```python
from build123d import *

# Parameters (mm, degrees)
BOSS_EXTRUDE1_DEPTH         = 12.7
BOSS_EXTRUDE1_DEPTH_BACK    = 12.7
SKETCH3_R                   = 69.85
SKETCH3_R_2                 = 57.15
CUT_EXTRUDE1_DEPTH          = 102.996102867
TAP_DRILL_FOR_1_4_20_TAP1_D = 5.1054
FILLET1_R                   = 2.54


with BuildPart() as part:
    # Sketch3 → Boss-Extrude1 (new, two sides: drawn at the far end of the back side and taken through both)
    with BuildSketch(Plane.XY.offset(-BOSS_EXTRUDE1_DEPTH_BACK)):
        Circle(SKETCH3_R)
        Circle(SKETCH3_R_2, mode=Mode.SUBTRACT)
    extrude(amount=BOSS_EXTRUDE1_DEPTH + BOSS_EXTRUDE1_DEPTH_BACK)

    # Sketch4 → Cut-Extrude1 (cut, through all)
    with BuildSketch(Plane.XY.offset(12.7)):
        with BuildLine():
            Line((-50.8, 69.120332123), (-50.8, -69.120332123))
            ThreePointArc((-50.8, -69.120332123), (85.780302592, 0), (-50.8, 69.120332123))
        make_face()
    extrude(amount=-CUT_EXTRUDE1_DEPTH, mode=Mode.SUBTRACT)

    # Tap Drill for 1/4-20 Tap1 (through all)
    with Locations(Plane.XY.offset(12.7)):
        with Locations((-57.15, -27.679008291), (-62.366515468, -11.944360527)):
            Hole(TAP_DRILL_FOR_1_4_20_TAP1_D / 2)

    # Fillet1
    fillet1_edges = [part.edges().sort_by_distance(p)[0] for p in [
        (-50.8, 47.941448664, 0),
        (-50.8, -47.941448664, 0),
    ]]
    fillet(fillet1_edges, radius=FILLET1_R)


solid = part.part
```
Input: part model. Units: mm. Frame: model coordinates. Give positions to 0.01 mm unless a question says otherwise; leave off trailing zeros. Loops run counter-clockwise (first coordinate to the right, second up) from the corner with the lowest first, then second, coordinate; pieces in that order, holes last.
1) Section query D-D on x = -68.25. Return the cut outline in (y, z), and give its area (3 significant figures).
A:
outline: (-14.86, -12.7) - (14.86, -12.7) - (14.86, 12.7) - (-14.86, 12.7) - close
area: 755 mm2
2) Line query: L1, parallel to Y at x = -61, z = 6.25; L2, parallel to Y at x = -57.5, z = -11.5; L3, parallel to X at y = 31.5, z = -11. Output: solid intervals per line, ascending.
A:
L1: y = -34.03 to -14.1, -9.79 to 34.03
L2: y = -39.66 to -30.21, -25.15 to 39.66
L3: x = -62.34 to -50.8
3) Contact query for flat-ended pins moving along their axis: pin 1 (1 mm diameter, centred on x = -64, z = 10, fed in from +Y); pin 2 (4.5 mm diameter, centred on x = -57.15, y = -27.68, fed in from -Z); pin 3 (10 mm diameter, centred on y = 27, z = -8.5, fed in from -X); pin 4 (3 mm diameter, centred on y = 4.5, z = -10, fed in from -X). Output: stop coordinate, or through.
A:
pin 1: stops at y = 29.1
pin 2: passes through
pin 3: stops at x = -66.29
pin 4: stops at x = -69.79
4) Mould query, pull axis Y, two halves, no side actions, for faces 1 (the flat face through (-50.8, -34, 0)), 2 (the cylindrical face through (-52.56, 43.47, -0.18)), 3 (the cylindrical face through (-57.15, 0.38, -0.18)). Classes: released by +Y, released by -Y, zero draft, split by the parting line, or undercut.
A:
face 1: zero draft
face 2: released by +Y
face 3: undercut
5) Section query B-B on z = -4.5. Return the cut outline in (x, y).
A:
outline: (-55.35, -42.6) arc R2.54 ccw to (-50.8, -41.05) - (-50.8, -26.18) arc R57.15 cw to (-50.8, 26.18) - (-50.8, 41.05) arc R2.54 ccw to (-55.35, 42.6) arc R69.85 ccw to start; hole circle Ø5.11 at (-62.37, -11.94); hole circle Ø5.11 at (-57.15, -27.68)
6) Section query C-C on y = -37. Return the cut outline in (x, z), and give its area (3 significant figures).
A:
outline: (-59.25, -12.7) - (-50.8, -12.7) - (-50.8, 12.7) - (-59.25, 12.7) - close
area: 215 mm2
7) Section query A-A on x = -56.25. Return the cut outline in (y, z), and give its area (3 significant figures).
A:
outline: (-41.41, -12.7) - (-30.07, -12.7) - (-30.07, 12.7) - (-41.41, 12.7) - close; (-25.29, -12.7) - (-10.1, -12.7) - (-10.1, 12.7) - (-25.29, 12.7) - close; (10.1, -12.7) - (41.41, -12.7) - (41.41, 12.7) - (10.1, 12.7) - close
area: 1,470 mm2
